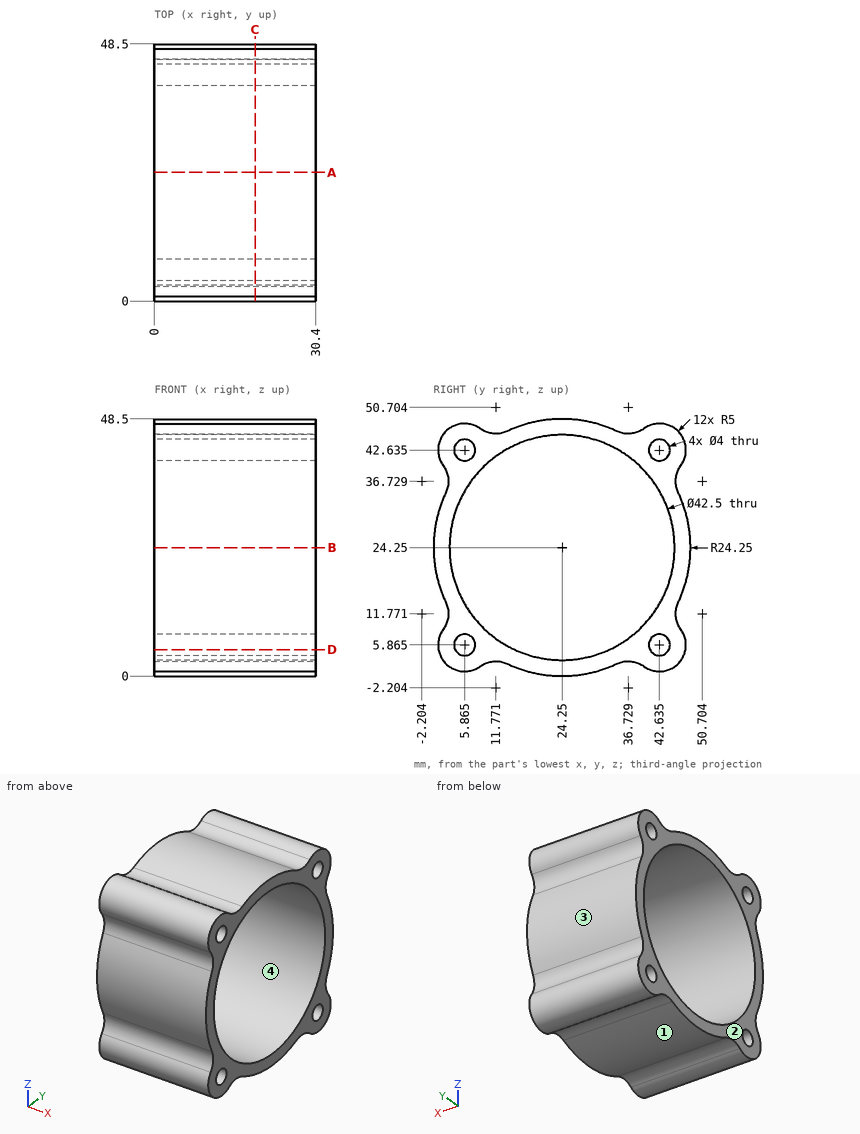
Verification items for this drawing (mm, ordinates from the low corner). Coordinates: 2 decimals unless noted, no trailing zeros. Order: outer loops, then holes, each group sorted by start corner. A loop starts at its lowest first (then second) coordinate and runs counter-clockwise, first axis right, second up. Notation, with made-up numbers: (39, 18) -> (91, 18) arc R23 cw to (91, 33) -> close; hole circle Ø3 at (16, 67.5). An arc over 180 degrees is marked (long way). Answer as CSV lines item,"result". Start each with the question number.
1) Cross-section at A-A, the plane y = 24.25. Record the boundary of the cut face in (x, z).
2) Cross-section at C-C, the plane x = 19. Give the number of separate pieces and of enclosed holes in the cut face, then the cut area to 3 significant figures.
3) Material ranges on L1, parallel to Y at x = 8.5, z = 24.25; L2, parallel to Y at x = 11, z = 41 (1 decimal); L3, parallel to Z at x = 2, y = 25, recorded low to high. Write a range as [from, to].
4) Release check for a two-part mould opening along Y. For the marked faces 1, 2, 3 and 4 record: released by +Y, released by -Y, zero draft, split by the parting line, or undercut.
5) Gauge pin test, flat ends, axial feed: pin 1 Ø1 at (x, y) = (10.5, 31.5) entering from +Z; pin 2 Ø3 at (x, y) = (8.5, 8) entering from +Z (1 decimal); pin 3 Ø1.5 at (x, y) = (23, 15) entering from -Z. Record the tip position at first contact, or that the pin passes through.
6) Cross-section at D-D, the plane z = 5. Record the boundary of the cut face in (x, y).
Conclusion:
1,outline,"(0, 0) -> (30.4, 0) -> (30.4, 3) -> (0, 3) -> close; (0, 45.5) -> (30.4, 45.5) -> (30.4, 48.5) -> (0, 48.5) -> close"
2,separate pieces,"1"
2,enclosed holes,"5"
2,area,"630 mm²"
3,L1,"y = [0, 3], [45.5, 48.5]"
3,L2,"y = [1.1, 4.7], [7, 11.2], [37.3, 41.5], [43.8, 47.4]"
3,L3,"z = [0.01, 3.01], [45.49, 48.49]"
4,face 1,"undercut"
4,face 2,"zero draft"
4,face 3,"released by +Y"
4,face 4,"undercut"
5,pin 1,"stops at z = 47.54"
5,pin 2,"stops at z = 47.6"
5,pin 3,"stops at z = 1.54"
6,outline,"(0, 0.94) -> (30.4, 0.94) -> (30.4, 4.06) -> (0, 4.06) -> close; (0, 7.67) -> (30.4, 7.67) -> (30.4, 15.25) -> (0, 15.25) -> close; (0, 33.25) -> (30.4, 33.25) -> (30.4, 40.83) -> (0, 40.83) -> close; (0, 44.44) -> (30.4, 44.44) -> (30.4, 47.56) -> (0, 47.56) -> close"
